Work out the finished part from the listing and answer in its coordinate system (mm). A direction names the side the tool comes from. Round coordinates to 2 decimals unless told otherwise and drop trailing zeros. Write each loop counter-clockwise with the first axis right and the second up, starting at its lowest first coordinate (ties: lowest second). Pieces come first, ordered by that corner, then holes. Notation, with made-up numbers: M 55.5,27 L 69.5,27 A28 ccw 69.5,53 Z; hole C -33,0.5 d3. An arc over 180 degrees is marked long. One line per item, written item: value. Start each with the question number.
Q1. Given pin 1 Ø8 at (x, z) = (350, 1.01) entering from +Y; pin 2 Ø3 at (x, z) = (57.61, 52.24) entering from -Y, each flat-ended and moving along its own axis, determine where each tip first touches the part or whether it passes through.
Q2. A tool of negligible diameter and unlimited length cuts with its end or side. For faces 1 (the cylindrical face through (80.27, 23.45, 92.58)), 2 (the flat face through (184, 0, -15)), 3 (the flat face through (184, 5, -11)), from which of +Z, -Z, +X, -X, +Y, -Y can it reach the whole face along a straight path? Write none if from no direction.
Q3. Find section C-C (x = 78). Write down the section's boundary in (y, z).
Q4. Consider probe 1 along X at (y, z) = (4, 117); probe 2 along Z at (x, y) = (350, 8); probe 3 along Z at (x, y) = (263, 1). Determine where each line is inside the solid, lowest interval first.
Q5. Find section B-B (z = 21.5). Write down the section's boundary in (x, y), and give its area (3 significant figures).
Q6. The mould has two halves that part along Z. Classify faces 4 (the flat face through (182, 10, 201.01)), 5 (the cylindrical face through (66.45, 13.69, 67.16)), 6 (the flat face through (182, 20, 89)): released by +Z, released by -Z, zero draft, split by the parting line, or undercut.
Q7. Find section D-D (z = 121.5). Write down the section's boundary in (x, y).
Q8. Find section A-A (x = 204). Write down the section's boundary in (y, z).
from build123d import *

# Parameters (mm, degrees)
SKETCH_2_W          = 370
SKETCH_2_H          = 220
EXTRUDE_1_DEPTH     = 20
SKETCH_3_R          = 2.5
CUT_EXTRUDE_1_DEPTH = 20
CUT_EXTRUDE_2_REACH = 423.551
SKETCH_4_R          = 35
SKETCH_5_R          = 45
EXTRUDE_2_DEPTH     = 7
SKETCH_6_R          = 35
CUT_EXTRUDE_3_DEPTH = 39
SKETCH_7_R          = 2.377872616
CUT_EXTRUDE_4_DEPTH = 39
CUT_EXTRUDE_5_DEPTH = 5


with BuildPart() as part:
    # 草图2 → 凸台-拉伸1 (new body)
    with BuildSketch(Plane(origin=(0, 0, 0), x_dir=(1, 0, 0), z_dir=(0, 1, 0))):
        with Locations((185, -91.010380349)):
            Rectangle(SKETCH_2_W, SKETCH_2_H)
    extrude(amount=EXTRUDE_1_DEPTH)

    # 草图3 → 切除-拉伸1 (cut)
    with BuildSketch(Plane(origin=(0, 20, 0), x_dir=(1, 0, 0), z_dir=(0, 1, 0))):
        with Locations(Location((15, 3.989619651, 0), (0, 0, 270))):
            Circle(SKETCH_3_R)
        with Locations(Location((20, -181.010380349, 0), (0, 0, 270))):
            Circle(SKETCH_3_R)
        with Locations(Location((350, -1.010380349, 0), (0, 0, 270))):
            Circle(SKETCH_3_R)
        with Locations(Location((350, -181.010380349, 0), (0, 0, 270))):
            Circle(SKETCH_3_R)
        with Locations(Location((180, -1.010380349, 0), (0, 0, 270))):
            Circle(SKETCH_3_R)
        with Locations(Location((180, -181.010380349, 0), (0, 0, 270))):
            Circle(SKETCH_3_R)
    extrude(amount=-CUT_EXTRUDE_1_DEPTH, mode=Mode.SUBTRACT)

    # 草图4 → 切除-拉伸2 (cut, up to next)
    with BuildSketch(Plane(origin=(0, 20, 0), x_dir=(1, 0, 0), z_dir=(0, 1, 0)), mode=Mode.PRIVATE) as cut_extrude_2_sk1:
        with Locations(Location((97.503107502, -51.010380349, 0), (0, 0, 270))):
            Circle(SKETCH_4_R)
    cut_extrude_2_tool1 = extrude(cut_extrude_2_sk1.sketch, amount=-CUT_EXTRUDE_2_REACH, mode=Mode.PRIVATE) & part.part
    add(cut_extrude_2_tool1.solids().sort_by_distance((97.503108, 20, 51.01038))[0], mode=Mode.SUBTRACT)

    # 草图5 → 凸台-拉伸2 (add)
    with BuildSketch(Plane(origin=(0, 20, 0), x_dir=(1, 0, 0), z_dir=(0, 1, 0))):
        with Locations(Location((97.503107502, -51.010380349, 0), (0, 0, 270))):
            Circle(SKETCH_5_R)
    extrude(amount=EXTRUDE_2_DEPTH)

    # 草图6 → 切除-拉伸3 (cut)
    with BuildSketch(Plane(origin=(0, 27, 0), x_dir=(1, 0, 0), z_dir=(0, 1, 0))):
        with Locations(Location((97.503107502, -51.010380349, 0), (0, 0, 270))):
            Circle(SKETCH_6_R)
    extrude(amount=-CUT_EXTRUDE_3_DEPTH, mode=Mode.SUBTRACT)

    # 草图7 → 切除-拉伸4 (cut)
    with BuildSketch(Plane(origin=(0, 27, 0), x_dir=(1, 0, 0), z_dir=(0, 1, 0))):
        with Locations(Location((96.273712382, -11.115523536, 0), (0, 0, 270))):
            Circle(SKETCH_7_R)
        with Locations(Location((137.397964314, -49.78098523, 0), (0, 0, 270))):
            Circle(SKETCH_7_R)
        with Locations(Location((98.732502621, -90.905237161, 0), (0, 0, 270))):
            Circle(SKETCH_7_R)
        with Locations(Location((57.608250689, -52.239775468, 0), (0, 0, 270))):
            Circle(SKETCH_7_R)
    extrude(amount=-CUT_EXTRUDE_4_DEPTH, mode=Mode.SUBTRACT)

    # 草图9 → 切除-拉伸5 (cut)
    with BuildSketch(Plane(origin=(0, 0, 0), x_dir=(-1, 0, 0), z_dir=(0, -1, 0))):
        with BuildLine():
            Line((-9.028166447, -196.169689035), (-360.428374593, -196.169689035))
            ThreePointArc((-360.428374593, -196.169689035), (-363.963908499, -194.705222941), (-365.428374593, -191.169689035))
            Line((-365.428374593, -191.169689035), (-365.428374593, 9.692387297))
            ThreePointArc((-365.428374593, 9.692387297), (-363.963908499, 13.227921203), (-360.428374593, 14.692387297))
            Line((-360.428374593, 14.692387297), (-9.028166447, 14.692387297))
            ThreePointArc((-9.028166447, 14.692387297), (-5.492632541, 13.227921203), (-4.028166447, 9.692387297))
            Line((-4.028166447, 9.692387297), (-4.028166447, -191.169689035))
            ThreePointArc((-4.028166447, -191.169689035), (-5.492632541, -194.705222941), (-9.028166447, -196.169689035))
        make_face()
        with BuildLine():
            Line((-12.832379165, -191.278558398), (-355.537243956, -191.278558398))
            ThreePointArc((-355.537243956, -191.278558398), (-359.072777862, -189.814092304), (-360.537243956, -186.278558398))
            Line((-360.537243956, -186.278558398), (-360.537243956, 4.257797701))
            ThreePointArc((-360.537243956, 4.257797701), (-359.072777862, 7.793331607), (-355.537243956, 9.257797701))
            Line((-355.537243956, 9.257797701), (-12.832379165, 9.257797701))
            ThreePointArc((-12.832379165, 9.257797701), (-9.296845259, 7.793331607), (-7.832379165, 4.257797701))
            Line((-7.832379165, 4.257797701), (-7.832379165, -186.278558398))
            ThreePointArc((-7.832379165, -186.278558398), (-9.296845259, -189.814092304), (-12.832379165, -191.278558398))
        make_face(mode=Mode.SUBTRACT)
    extrude(amount=-CUT_EXTRUDE_5_DEPTH, mode=Mode.SUBTRACT)


solid = part.part
The answers:
1. pin 1: y = 20
1. pin 2: through
2. face 1: +Y
2. face 2: +Z, -Z, +X, -X, -Y
2. face 3: -Y
3. outline: M 0,-18.99 L 20,-18.99 L 20,10.46 L 27,10.46 L 27,21.95 L 0,21.95 L 0,-9.26 L 5,-9.26 L 5,-14.69 L 0,-14.69 Z; M 0,80.07 L 27,80.07 L 27,91.56 L 20,91.56 L 20,201.01 L 0,201.01 L 0,196.17 L 5,196.17 L 5,191.28 L 0,191.28 Z
4. probe 1: 0 to 4.03, 7.83 to 360.54, 365.43 to 370
4. probe 2: -18.99 to -1.49, 3.51 to 178.51, 183.51 to 201.01
4. probe 3: -18.99 to -14.69, -9.26 to 191.28, 196.17 to 201.01
5. outline: M 0,0 L 4.03,0 L 4.03,5 L 7.83,5 L 7.83,0 L 78.68,0 L 78.68,27 L 63.53,27 L 63.53,20 L 0,20 Z; M 116.32,0 L 360.54,0 L 360.54,5 L 365.43,5 L 365.43,0 L 370,0 L 370,20 L 131.48,20 L 131.48,27 L 116.32,27 Z
5. area: 6,820 mm2
6. face 4: released by +Z
6. face 5: undercut
6. face 6: zero draft
7. outline: M 0,0 L 4.03,0 L 4.03,5 L 7.83,5 L 7.83,0 L 360.54,0 L 360.54,5 L 365.43,5 L 365.43,0 L 370,0 L 370,20 L 0,20 Z
8. outline: M 0,-18.99 L 20,-18.99 L 20,201.01 L 0,201.01 L 0,196.17 L 5,196.17 L 5,191.28 L 0,191.28 L 0,-9.26 L 5,-9.26 L 5,-14.69 L 0,-14.69 Z
